```python
from build123d import *

# Parameters (mm, degrees)
F1_DEPTH = 3
F2_W     = 3
F2_H     = 734
F3_DEPTH = 10


with BuildPart() as f1:
    # F0 (on Right) → F1 (new body)
    with BuildSketch(Plane.YZ):
        Polygon((-400, 0), (0, 0), (0, 160), (-230, 160), (-230, 850), (-370, 1000), (-400, 1000), align=None)
    extrude(amount=F1_DEPTH)

    # F2 (on face) → F3 (join)
    with BuildSketch(Plane.YZ.offset(3)):
        with Locations((-398.5, 633)):
            Rectangle(F2_W, F2_H)
    extrude(amount=F3_DEPTH)


solid = f1.part
```
Geometry check sheet. Reference: the model listing, model coordinates, mm. Round coordinates to 2 decimals unless told otherwise and drop trailing zeros. Order: outer loops, then holes, each group sorted by start corner. A loop starts at its lowest first (then second) coordinate and runs counter-clockwise, first axis right, second up. Notation, with made-up numbers: (21.25, 7) - (78.25, 7) arc R19 cw to (78.25, 44) - close; hole circle Ø6 at (78, 25). An arc over 180 degrees is marked (long way). Use a Markdown table: item, result. Add a question column.
(1) Sectioned sample at B-B, the plane z = 884.5. Enter the section's corners in (x, y), and give its area (3 significant figures).
(2) Sectioned sample at A-A, the plane x = 9.25. Enter the section's corners in (y, z).
(3) Sectioned sample at D-D, the plane z = 294. Enter the section's corners in (x, y), and give its area (3 significant figures).
(4) Material ranges on line 1 along Y through (x, z) = (9.75, 468.5); line 2 along X through (y, z) = (-167, 136), recorded low to high. Write a range as [from, to].
(5) Depth check by flat-ended pin: pin 1 (2.5 mm diameter, centred on x = 9.5, y = -399, fed in from -Z); pin 2 (3.5 mm diameter, centred on x = 1.5, z = 649, fed in from +Y); pin 3 (6 mm diameter, centred on y = -312.5, z = 515.5, fed in from +X). Enter the tip coordinate at first touch or a pass-through.
(6) Sectioned sample at C-C, the plane y = -356. Enter the section's corners in (x, z), and give its area (4 significant figures).
Answers below:
| question | item | result |
|---|---|---|
| 1 | outline | (0, -400) - (13, -400) - (13, -397) - (3, -397) - (3, -262.2) - (0, -262.2) - close |
| 1 | area | 443 mm² |
| 2 | outline | (-400, 266) - (-397, 266) - (-397, 1000) - (-400, 1000) - close |
| 3 | outline | (0, -400) - (13, -400) - (13, -397) - (3, -397) - (3, -230) - (0, -230) - close |
| 3 | area | 540 mm² |
| 4 | line 1 | [-400, -397] |
| 4 | line 2 | [0, 3] |
| 5 | pin 1 | z = 266 |
| 5 | pin 2 | y = -230 |
| 5 | pin 3 | x = 3 |
| 6 | outline | (0, 0) - (3, 0) - (3, 985) - (0, 985) - close |
| 6 | area | 2,955 mm² |
